Here's how the part is built. I have some questions about the finished solid (model axes, mm). Face numbers are marked on the shaded views. A direction names the side the tool comes from. Give positions to 0.01 mm unless a question says otherwise; leave off trailing zeros. Order: outer loops, then holes, each group sorted by start corner. A loop starts at its lowest first (then second) coordinate and runs counter-clockwise, first axis right, second up. Notation, with made-up numbers: M 73,83 L 111,83 A24 ccw 111,109 Z; hole C 65,-33 d7. An arc over 180 degrees is marked long. Use one line per item in the form item = value.
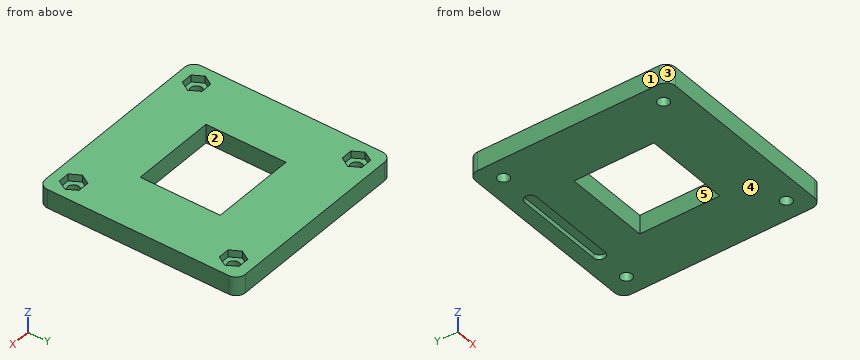
from build123d import *

# Parameters (mm, degrees)
SKETCH1_R           = 1.2
SKETCH1_W           = 18.2
SKETCH1_H           = 17
BOSS_EXTRUDE1_DEPTH = 4
CUT_EXTRUDE3_DEPTH  = 1
CUT_EXTRUDE4_DEPTH  = 1.5


with BuildPart() as part:
    # Sketch1 → Boss-Extrude1 (new body)
    with BuildSketch(Plane.XY):
        with BuildLine():
            Line((21.25, -19.25), (21.25, 19.25))
            ThreePointArc((21.25, 19.25), (20.664213562, 20.664213562), (19.25, 21.25))
            Line((19.25, 21.25), (-19.25, 21.25))
            ThreePointArc((-19.25, 21.25), (-20.664213562, 20.664213562), (-21.25, 19.25))
            Line((-21.25, 19.25), (-21.25, -19.25))
            ThreePointArc((-21.25, -19.25), (-20.664213562, -20.664213562), (-19.25, -21.25))
            Line((-19.25, -21.25), (19.25, -21.25))
            ThreePointArc((19.25, -21.25), (20.664213562, -20.664213562), (21.25, -19.25))
        make_face()
        with Locations((-17, -17)):
            Circle(SKETCH1_R, mode=Mode.SUBTRACT)
        with Locations((17, -17)):
            Circle(SKETCH1_R, mode=Mode.SUBTRACT)
        with Locations((17, 17)):
            Circle(SKETCH1_R, mode=Mode.SUBTRACT)
        with Locations((-17, 17)):
            Circle(SKETCH1_R, mode=Mode.SUBTRACT)
        with Locations((0, -0.4)):
            Rectangle(SKETCH1_W, SKETCH1_H, mode=Mode.SUBTRACT)
    extrude(amount=BOSS_EXTRUDE1_DEPTH)

    # Sketch2 → Cut-Extrude3 (cut)
    with BuildSketch(Plane(origin=(0, 0, 0), x_dir=(-1, 0, 0), z_dir=(0, 0, -1))):
        with BuildLine():
            Line((-9.5, 18.25), (9.5, 18.25))
            ThreePointArc((9.5, 18.25), (10.75, 17), (9.5, 15.75))
            Line((9.5, 15.75), (-9.5, 15.75))
            ThreePointArc((-9.5, 15.75), (-10.75, 17), (-9.5, 18.25))
        make_face()
    extrude(amount=-CUT_EXTRUDE3_DEPTH, mode=Mode.SUBTRACT)

    # Sketch3 → Cut-Extrude4 (cut)
    with BuildSketch(Plane.XY.offset(4)):
        Polygon((-18.212435565, -14.9), (-19.424871131, -17), (-18.212435565, -19.1), (-15.787564435, -19.1), (-14.575128869, -17), (-15.787564435, -14.9), align=None)
        Polygon((15.787564435, -14.9), (14.575128869, -17), (15.787564435, -19.1), (18.212435565, -19.1), (19.424871131, -17), (18.212435565, -14.9), align=None)
        Polygon((-18.212435565, 19.1), (-19.424871131, 17), (-18.212435565, 14.9), (-15.787564435, 14.9), (-14.575128869, 17), (-15.787564435, 19.1), align=None)
        Polygon((15.787564435, 19.1), (14.575128869, 17), (15.787564435, 14.9), (18.212435565, 14.9), (19.424871131, 17), (18.212435565, 19.1), align=None)
    extrude(amount=-CUT_EXTRUDE4_DEPTH, mode=Mode.SUBTRACT)


solid = part.part
Q1. Thinking about a two-plate mould opening in Y: for the marked faces 3, 4 and 5, which applies, +Y half, -Y half, draft (parallel to the pull), parting line (faces both ways), or undercut?
Found:
face_3 = -Y half
face_4 = draft
face_5 = undercut
Q2. I want a section at D-D on x = 17. Write out the boundary of the cut face in (y, z).
Found:
outline = M -21.25,0 L -18.2,0 L -18.2,2.5 L -19.1,2.5 L -19.1,4 L -21.25,4 Z; M -15.8,0 L 15.8,0 L 15.8,2.5 L 14.9,2.5 L 14.9,4 L -14.9,4 L -14.9,2.5 L -15.8,2.5 Z; M 18.2,0 L 21.25,0 L 21.25,4 L 19.1,4 L 19.1,2.5 L 18.2,2.5 Z
Q3. I want a section at A-A on y = 0.5. Write out the boundary of the cut face in (x, z), then the cut area to 3 significant figures.
Found:
outline = M -21.25,0 L -9.1,0 L -9.1,4 L -21.25,4 Z; M 9.1,0 L 21.25,0 L 21.25,4 L 9.1,4 Z
area = 97.2 mm²
Q4. I want a section at C-C on z = 2. Write out the boundary of the cut face in (x, y).
Found:
outline = M -21.25,-19.25 A2 ccw -19.25,-21.25 L 19.25,-21.25 A2 ccw 21.25,-19.25 L 21.25,19.25 A2 ccw 19.25,21.25 L -19.25,21.25 A2 ccw -21.25,19.25 Z; hole C -17,-17 d2.4; hole C -17,17 d2.4; hole M -9.1,-8.9 L 9.1,-8.9 L 9.1,8.1 L -9.1,8.1 Z; hole C 17,-17 d2.4; hole C 17,17 d2.4
Q5. I want a section at B-B on x = -5.5. Write out the boundary of the cut face in (y, z).
Found:
outline = M -21.25,0 L -8.9,0 L -8.9,4 L -21.25,4 Z; M 8.1,0 L 15.75,0 L 15.75,1 L 18.25,1 L 18.25,0 L 21.25,0 L 21.25,4 L 8.1,4 Z
Q6. I need wall thicknesses on L1, parallel to X at y = 17, z = 0.8; L2, parallel to X at y = -17, z = 0.75. Which ranges of each line are inside material? Lowest first, please.
Found:
L1 = -21.25 to -18.2, -15.8 to -10.75, 10.75 to 15.8, 18.2 to 21.25
L2 = -21.25 to -18.2, -15.8 to 15.8, 18.2 to 21.25
Q7. On a 3-axis mill with a long thin cutter (end or side, diameter ignored), from which of +Z, -Z, +X, -X, +Y, -Y can I reach the whole of each face in a straight line? I mean the marked faces 1 and 2. Say none if no direction works.
Found:
face_1 = +Z, -Z, -X, +Y, -Y
face_2 = +Z, -Z
Q8. I'm going to push flat-ended pins straight in: pin 1 Ø3 at (x, y) = (-17, -17) entering from -Z; pin 2 Ø2 at (x, y) = (-17, -17.5) entering from +Z. Where does each tip first touch, or does it pass through?
Found:
pin_1 = 0
pin_2 = 2.5
